Source: CAD feature listing. Evaluate the final solid. Frame: model axes, mm. Face numbers are marked on the shaded views. A direction names the side the tool comes from. Round coordinates to 2 decimals unless told otherwise and drop trailing zeros. Loops run counter-clockwise (first coordinate to the right, second up) from the corner with the lowest first, then second, coordinate; pieces in that order, holes last.
(1) Set-up query: the marked faces 1, 2 and 3. Return all of +Z, -Z, +X, -X, +Y, -Y with unobstructed straight access to the full face (end or side cutting, diameter ignored); none if empty.
(2) Section B-B, the plane x = -6.5. Return the cut outline in (y, z), plus the area to 3 significant figures.
(3) Section C-C, the plane y = -0.5. Return the cut outline in (x, z).
(4) Section A-A, the plane y = -49.15. Return the cut outline in (x, z) (3 decimals), plus the area to 3 significant figures.
(5) Section D-D, the plane y = 12. Return the cut outline in (x, z).
(6) Mould query, pull axis Y, two halves, no side actions, for the marked faces 4, 5 and 6. Classes: pulls with the +Y half, pulls with the -Y half, needs draft (parallel to the pull), parting line crosses it, or undercut.
(7) Material intervals for probe 1 along X at (y, z) = (-49.15, 1.9) (3 decimals); probe 2 along Y at (x, z) = (-18.5, 7); probe 3 along Y at (x, z) = (-6.5, 4), sorted ascending.
(8) First-contact query: pin 1 Ø5 at (x, y) = (0.5, 50) entering from +Z; pin 2 Ø5 at (y, z) = (50, 6.5) entering from +X; pin 3 Ø2 at (y, z) = (26.5, 6.5) entering from +X; pin 4 Ø2 at (x, y) = (21.975, -49.15) entering from -Z. Flat tips, straight axial feed; report the tip coordinate or a pass-through.
Autodesk Inventor part; units mm, degrees
ref_plane "YZ Plane" through (0, 0, 0) normal (1, 0, 0) x (0, 1, 0)
ref_plane "XZ Plane" through (0, 0, 0) normal (0, 1, 0) x (-1, 0, 0)
ref_plane "XY Plane" through (0, 0, 0) normal (0, 0, 1) x (1, 0, 0)
sketch "Boceto1" plane through (0, 0, 0) normal (0, 0, 1) x (1, 0, 0)
  line L0 (27.55, -53.55) -> (-27.55, -53.55)
  line L1 (-27.55, -53.55) -> (-27.55, 53.55)
  line L2 (-27.55, 53.55) -> (27.55, 53.55)
  line L3 (27.55, 53.55) -> (27.55, -53.55)
  line L4 (27.55, -53.55) -> (-27.55, 53.55) construction
  line L5 (-27.55, -53.55) -> (27.55, 53.55) construction
  line L6 (20.325, -47.5) -> (-20.325, -47.5)
  line L7 (-20.325, -47.5) -> (-20.325, 47.5)
  line L8 (-20.325, 47.5) -> (20.325, 47.5)
  line L9 (20.325, 47.5) -> (20.325, -47.5)
  line L10 (20.325, -47.5) -> (-20.325, 47.5) construction
  line L11 (-20.325, -47.5) -> (20.325, 47.5) construction
  line L12 (-20.325, 47.5) -> (-21.975, 47.5)
  line L13 (-21.975, 47.5) -> (-21.975, 49.15)
  line L14 (-21.975, 49.15) -> (-21.975, -49.15)
  line L15 (-21.975, -49.15) -> (21.975, -49.15)
  line L16 (21.975, -49.15) -> (21.975, 49.15)
  line L17 (21.975, 49.15) -> (-21.975, 49.15)
  circle A0 centre (-21.975, 49.15) radius 1.65
  circle A1 centre (21.975, 49.15) radius 1.65
  circle A2 centre (21.975, -49.15) radius 1.65
  circle A3 centre (-21.975, -49.15) radius 1.65
  point P0 (0, 0)
  point P1 (20.325, 49.15)
  point P2 (21.975, 47.5)
  dimension "d0" = 55.1
  dimension "d1" = 107.1
  dimension "d2" = 40.65
  dimension "d3" = 95
  dimension "d4" = 1.65
  dimension "d5" = 1.65
  dimension "d6" = 1.65
  dimension "d7" = 3.3
  dimension "d8" = 3.3
  dimension "d9" = 3.3
extrude "Extrusión1" add sketch "Boceto1" along normal blind 16.35 contours L0 L1 L2 L3 | A0 L17 A1 L16 A2 L15 A3 L14 | L6 L7 L8 L9 | L17 L16 A1 picked at (20.8888, 49.0276)
sketch "Boceto2" plane through (-27.55, -53.55, 0) normal (-1, 0, 0) x (0, 0, 1)
  line L0 (0, 107.1) -> (0, 88.8)
  line L1 (0, 107.1) -> (0, 0)
  line L2 (0, 107.1) -> (3.3, 107.1)
  line L3 (3.3, 107.1) -> (3.3, 53.55)
  line L4 (3.3, 53.55) -> (3.3, 0)
  line L5 (0, 0) -> (16.35, 0)
  line L6 (3.3, 107.1) -> (11.9, 107.1)
  line L7 (0, 107.1) -> (16.35, 107.1)
  line L8 (11.9, 107.1) -> (11.9, 101.1)
  line L9 (11.9, 101.1) -> (3.3, 101.1)
  line L10 (3.3, 107.1) -> (3.3, 89.1)
  line L11 (0, 102.7) -> (16.35, 102.7)
  line L12 (3.3, 107.1) -> (21.3, 107.1) construction
  line L13 (3.3, 89.1) -> (10, 89.1)
  line L14 (10, 89.1) -> (10, 73.1)
  line L15 (10, 73.1) -> (3.3, 73.1)
  line L16 (3.3, 107.1) -> (3.3, 59.9)
  line L17 (3.3, 59.9) -> (16.3, 59.9)
  line L18 (16.3, 59.9) -> (16.35, 59.9)
  line L19 (16.35, 107.1) -> (16.35, 0)
  line L20 (16.35, 59.9) -> (16.35, 29.8)
  line L21 (16.35, 59.9) -> (46.45, 59.9) construction
  line L22 (16.35, 29.8) -> (3.3, 29.8)
  line L23 (3.3, 0) -> (3.3, 6.2)
  line L24 (3.3, 6.2) -> (14.8, 6.2)
  line L25 (16.35, 6.05) -> (0, 6.05)
  line L26 (3.3, 6.2) -> (14.8, 6.2) construction
  line L27 (14.8, 6.2) -> (14.8, 15.2)
  line L28 (14.8, 6.2) -> (23.8, 6.2) construction
  line L29 (14.8, 15.2) -> (3.3, 15.2)
  line L30 (3.3, 0) -> (3.3, 20)
  line L31 (3.3, 0) -> (23.3, 0) construction
  line L32 (3.3, 20) -> (12.6, 20)
  line L33 (12.6, 20) -> (12.6, 27.2)
  line L34 (12.6, 27.2) -> (3.3, 27.2)
  point P0 (0, 53.55)
  dimension "d17" = 3.3
  dimension "d18" = 8.6
  dimension "d19" = 6
  dimension "d20" = 18
  dimension "d21" = 90
  dimension "d22" = 6.7
  dimension "d23" = 16
  dimension "d24" = 47.2
  dimension "d25" = 13
  dimension "d26" = 90
  dimension "d27" = 30.1
  dimension "d28" = 90
  dimension "d29" = 6.2
  dimension "d30" = 11.5
  dimension "d31" = 0
  dimension "d32" = 9
  dimension "d33" = 90
  dimension "d34" = 20
  dimension "d35" = 90
  dimension "d36" = 9.3
  dimension "d37" = 90
  dimension "d38" = 7.2
  dimension "d39" = 90
extrude "Extrusión2" cut sketch "Boceto2" against normal through all contours L7 L19 L11 L8 | L9 L8 L11 L19 L18 L17 L3 L15 L14 L13 | L25 L19 L5 L4 | L4 L24 L27 L29 L32 L33 L34 L22 L19 L25
sketch "Boceto3" plane through (0, 0, 16.35) normal (0, 0, 1) x (1, 0, 0)
  line L0 (-27.55, 53.55) -> (27.55, 53.55)
  line L1 (27.55, 47.55) -> (27.55, 35.55)
  line L2 (27.55, 53.55) -> (27.55, 47.55)
  line L3 (27.55, 35.55) -> (27.55, 19.55)
  line L4 (27.55, 19.55) -> (27.55, 6.35)
  line L5 (27.55, -23.75) -> (27.55, 6.35)
  line L6 (27.55, -26.35) -> (27.55, -33.55)
  line L7 (-27.55, 53.55) -> (-27.55, -53.55)
  line L8 (27.55, 53.55) -> (-27.55, 53.55)
  line L9 (-27.55, -53.55) -> (27.55, -53.55)
  line L10 (27.55, -53.55) -> (27.55, 53.55)
  line L11 (-27.55, 53.55) -> (-13.45, 53.55)
  line L12 (-21.5719, 47.55) -> (21.975, 47.55)
  line L13 (-27.55, 35.55) -> (27.55, 35.55)
  line L14 (-27.55, 19.55) -> (27.55, 19.55)
  line L15 (-27.55, 6.35) -> (27.55, 6.35)
  line L16 (-27.55, -23.75) -> (27.55, -23.75)
  line L17 (-27.55, -26.35) -> (27.55, -26.35)
  line L18 (-27.55, -33.55) -> (27.55, -33.55)
  line L19 (-27.55, -38.35) -> (27.55, -38.35)
  line L20 (27.55, -38.35) -> (27.55, -47.35)
  line L21 (-27.55, -38.35) -> (27.55, -38.35)
  line L22 (-27.55, -47.35) -> (-27.55, -38.35)
  line L23 (-27.55, -47.35) -> (27.55, -47.35)
  line L24 (27.55, -47.35) -> (27.55, -53.55)
  line L25 (-27.55, -47.35) -> (27.55, -47.35)
  line L26 (-27.55, -53.55) -> (-27.55, -47.35)
  line L27 (27.55, -53.55) -> (-27.55, -53.55)
  circle A0 centre (-21.975, -49.15) radius 1.65
  circle A1 centre (21.975, -49.15) radius 1.65
  line L28 (27.55, 53.55) -> (-27.55, 53.55)
  line L29 (27.55, 53.55) -> (27.55, 47.55)
  line L30 (-27.55, 53.55) -> (27.55, 53.55)
  line L31 (-27.55, 47.55) -> (-27.55, 53.55)
  line L32 (-27.55, 47.55) -> (-22.3781, 47.55)
  arc A2 (-21.5719, 47.55) -> (-22.3781, 47.55) centre (-21.975, 49.15) ccw
  line L33 (-21.5719, 47.55) -> (21.975, 47.55)
  line L34 (21.975, 49.15) -> (21.975, 47.55)
  line L35 (20.325, 49.15) -> (21.975, 49.15)
  arc A3 (22.3781, 47.55) -> (20.325, 49.15) centre (21.975, 49.15) ccw
  line L36 (22.3781, 47.55) -> (27.55, 47.55)
  line L37 (-13.45, 53.55) -> (-13.45, 47.55)
  line L38 (27.55, 53.55) -> (8.75, 53.55)
  line L39 (8.75, 53.55) -> (8.75, 47.55)
  line L40 (-21.5719, 47.55) -> (21.975, 47.55)
  line L41 (-27.55, 35.55) -> (-27.55, 47.55)
  line L42 (-27.55, 35.55) -> (-15.55, 35.55)
  line L43 (-15.55, 35.55) -> (-15.55, 19.55)
  line L44 (27.55, 6.35) -> (-27.55, 6.35)
  line L45 (-27.55, 6.35) -> (-18.15, 6.35)
  line L46 (-18.15, 6.35) -> (-18.15, -26.35)
  line L47 (-27.55, -26.35) -> (-1.55, -26.35)
  line L48 (-1.55, -26.35) -> (-1.55, -33.55)
  line L49 (-27.55, -38.35) -> (-12.55, -38.35)
  line L50 (-12.55, -38.35) -> (-12.55, -47.35)
  point P0 (0, 0)
  point P1 (-18.15, -23.75)
  point P2 (21.975, 47.55)
  dimension "d42" = 14.1
  dimension "d43" = 18.8
  dimension "d44" = 12
  dimension "d45" = 9.4
  dimension "d46" = 26
  dimension "d47" = 15
extrude "Extrusión3" cut sketch "Boceto3" against normal up to surface (13.05 mm away) contours L0 L37 L12 A2 L32 L7 | L0 L2 L36 A3 L35 L34 L12 L39 | L13 L3 L14 L43 | L15 L5 L16 L46 | L48 L17 L6 L18 | L19 L10 L23 L50
properties part number "placa"
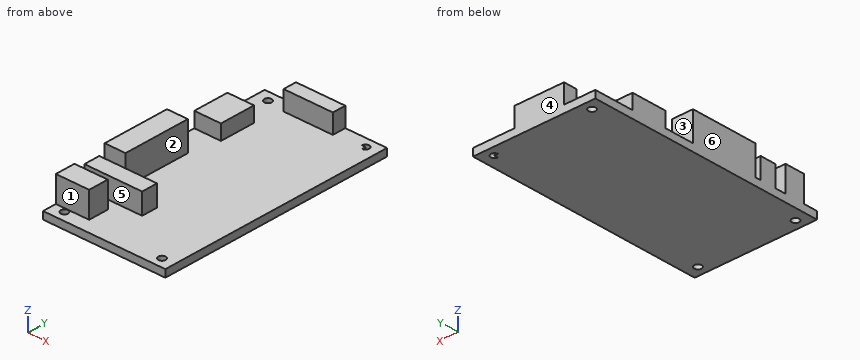
Output values:
1. face 1: +Z, +X, -X, -Y
1. face 2: +Z, +X
1. face 3: +Z, +X, -X
2. outline: (-53.55, 0) - (53.55, 0) - (53.55, 11.9) - (47.55, 11.9) - (47.55, 3.3) - (-26.35, 3.3) - (-26.35, 12.6) - (-33.55, 12.6) - (-33.55, 3.3) - (-53.55, 3.3) - close
2. area: 472 mm2
3. outline: (-27.55, 0) - (27.55, 0) - (27.55, 3.3) - (-18.15, 3.3) - (-18.15, 16.35) - (-27.55, 16.35) - close
4. outline: (-27.55, 0) - (-23.625, 0) - (-23.625, 3.3) - (-27.55, 3.3) - close; (-20.325, 0) - (20.325, 0) - (20.325, 3.3) - (-20.325, 3.3) - close; (23.625, 0) - (27.55, 0) - (27.55, 3.3) - (23.625, 3.3) - close
4. area: 160 mm2
5. outline: (-27.55, 0) - (27.55, 0) - (27.55, 3.3) - (-27.55, 3.3) - close
6. face 4: pulls with the +Y half
6. face 5: undercut
6. face 6: needs draft
7. probe 1: x = -27.55 to -23.625, -20.325 to 20.325, 23.625 to 27.55
7. probe 2: y = -47.35 to -38.35, -33.55 to -26.35, -23.75 to 6.35, 19.55 to 35.55
7. probe 3: y = -33.55 to -26.35, 47.55 to 53.55
8. pin 1: stops at z = 11.9
8. pin 2: stops at x = 8.75
8. pin 3: stops at x = -15.55
8. pin 4: passes through
